```python
from build123d import *

# Parameters (mm, degrees)
SKETCH_1_W          = 6.2
SKETCH_1_H          = 6.2
SKETCH_1_R          = 1.2
EXTRUDE_1_DEPTH     = 2
CUT_EXTRUDE_1_DEPTH = 1
SKETCH_3_W          = 10
SKETCH_3_H          = 12.5
CUT_EXTRUDE_2_DEPTH = 1
CHAMFER_1_SIZE      = 1
SKETCH_4_W          = 44.4
SKETCH_4_H          = 18.5
SKETCH_4_W_2        = 38.4
SKETCH_4_H_2        = 12.5
EXTRUDE_2_DEPTH     = 3
CHAMFER_2_SIZE      = 2


with BuildPart() as part:
    # 草图1 → 凸台-拉伸1 (new body)
    with BuildSketch(Plane.XY):
        Polygon((-68.63, 16.2), (-64.63, 12.2), (-64.63, -37.62), (-68.63, -41.62), (-68.63, -49.62), (11.17, -49.62), (11.17, -41.62), (7.17, -37.62), (7.17, 12.2), (11.17, 16.2), (11.17, 38.1), (-68.63, 38.1), align=None)
        with Locations((-37.93, 28.38)):
            Rectangle(SKETCH_1_W, SKETCH_1_H, mode=Mode.SUBTRACT)
        with Locations((-27.73, 28.38)):
            Rectangle(SKETCH_1_W, SKETCH_1_H, mode=Mode.SUBTRACT)
        with Locations((-66.63, -45.62)):
            Circle(SKETCH_1_R, mode=Mode.SUBTRACT)
        with Locations((9.17, -45.62)):
            Circle(SKETCH_1_R, mode=Mode.SUBTRACT)
        with Locations((-66.63, 20.2)):
            Circle(SKETCH_1_R, mode=Mode.SUBTRACT)
        with Locations((9.17, 20.2)):
            Circle(SKETCH_1_R, mode=Mode.SUBTRACT)
    extrude(amount=EXTRUDE_1_DEPTH)

    # 草图2 → 切除-拉伸1 (cut)
    with BuildSketch(Plane.XY.offset(2)):
        Polygon((-12.23, -27.12), (-39.83, -27.12), (-39.83, -35.02), (-39.83, -39.62), (-12.23, -39.62), align=None)
        Polygon((-39.83, -27.12), (-50.63, -27.12), (-50.63, -39.62), (-39.83, -39.62), (-39.83, -35.02), align=None)
    extrude(amount=-CUT_EXTRUDE_1_DEPTH, mode=Mode.SUBTRACT)

    # 草图3 → 切除-拉伸2 (cut)
    with BuildSketch(Plane.XY.offset(1)):
        with Locations((-45.63, -33.37)):
            Rectangle(SKETCH_3_W, SKETCH_3_H)
    extrude(amount=-CUT_EXTRUDE_2_DEPTH, mode=Mode.SUBTRACT)

    # 倒角1
    chamfer_1_edges = [part.edges().sort_by_distance(p)[0] for p in [
        (-37.93, 25.28, 2),
        (-41.03, 28.38, 2),
        (-37.93, 31.48, 2),
        (-27.73, 31.48, 2),
        (-24.63, 28.38, 2),
        (-27.73, 25.28, 2),
        (-30.83, 28.38, 2),
        (-34.83, 28.38, 2),
    ]]
    chamfer(chamfer_1_edges, length=CHAMFER_1_SIZE)

    # 草图4 → 凸台-拉伸2 (add)
    with BuildSketch(Plane.XY.offset(2)):
        with Locations((-31.43, -33.37)):
            Rectangle(SKETCH_4_W, SKETCH_4_H)
        with Locations((-31.43, -33.37)):
            Rectangle(SKETCH_4_W_2, SKETCH_4_H_2, mode=Mode.SUBTRACT)
    extrude(amount=EXTRUDE_2_DEPTH)

    # 倒角2
    chamfer_2_edges = [part.edges().sort_by_distance(p)[0] for p in [
        (-31.43, -24.12, 5),
        (-9.23, -33.37, 5),
        (-53.63, -33.37, 5),
        (-31.43, -42.62, 5),
    ]]
    chamfer(chamfer_2_edges, length=CHAMFER_2_SIZE)


solid = part.part
```
Check sheet for the modelled part. Datum: model origin and axes. Units: mm. A direction names the side the tool comes from. Round coordinates to 2 decimals unless told otherwise and drop trailing zeros. Order: outer loops, then holes, each group sorted by start corner. A loop starts at its lowest first (then second) coordinate and runs counter-clockwise, first axis right, second up.
1) Go/stop test with flat-tipped pins: pin 1 Ø1 at (y, z) = (1, 4) entering from -X; pin 2 Ø1.6 at (y, z) = (-4.5, 1.5) entering from +X; pin 3 Ø0.5 at (x, z) = (-41, 2.5) entering from -Y; pin 4 Ø3 at (x, y) = (-66.63, 20.2) entering from +Z. Record where each tip stops, or that it passes through.
2) Section check A-A (y = -45.62). Record the boundary of the cut face in (x, z), and give its area (3 significant figures).
3) Scan lines: line 1 (Y direction, x = -21.5, z = 1.25); line 2 (Y direction, x = -66.63, z = 1.2); line 3 (X direction, y = -36.5, z = 0.35). Record each from-to range of solid material in increasing order.
4) Section check D-D (y = 26.5). Record the boundary of the cut face in (x, z).
5) Mould release check, pull along X, two halves, no side actions. Record for faces 1 (the cylindrical face through (9.724, -46.685, 0.986)), 2 (the flat face through (11.17, -46, 1)), 3 (the flat face through (-68.63, -46, 1)), 4 (the flat face through (-31.74, -25.11, 3.99)): +X half, -X half, draft (parallel to the pull), parting line (faces both ways), or undercut.
6) Section check B-B (x = -48). Record the boundary of the cut face in (y, z), and give its area (3 significant figures).
7) Section check C-C (x = -66.63). Record the boundary of the cut face in (y, z).
8) Tool access check on faces 5 (the flat face through (-64.63, -12, 1)), 6 (the flat face through (-27, -33, 1)), 7 (the flat face through (7.17, -13, 1)), 8 (the flat face through (-50.63, -33, 2)). Record the directions out of +Z, -Z, +X, -X, +Y, -Y that give a thin tool (end or side, any length) a straight path to the whole face; none if there is none.
Result:
1. pin 1: passes through
1. pin 2: stops at x = 7.17
1. pin 3: stops at y = -42.62
1. pin 4: stops at z = 2
2. outline: (-68.63, 0) - (-67.83, 0) - (-67.83, 2) - (-68.63, 2) - close; (-65.43, 0) - (7.97, 0) - (7.97, 2) - (-65.43, 2) - close; (10.37, 0) - (11.17, 0) - (11.17, 2) - (10.37, 2) - close
2. area: 150 mm2
3. line 1: y = -49.62 to -39.62, -27.12 to 38.1
3. line 2: y = -49.62 to -46.82, -44.42 to -39.62, 14.2 to 19, 21.4 to 38.1
3. line 3: x = -64.63 to -50.63, -40.63 to 7.17
4. outline: (-68.63, 0) - (-41.03, 0) - (-41.03, 1) - (-42.03, 2) - (-68.63, 2) - close; (-34.83, 0) - (-30.83, 0) - (-30.83, 1) - (-31.83, 2) - (-33.83, 2) - (-34.83, 1) - close; (-24.63, 0) - (11.17, 0) - (11.17, 2) - (-23.63, 2) - (-24.63, 1) - close
5. face 1: undercut
5. face 2: +X half
5. face 3: -X half
5. face 4: draft
6. outline: (-49.62, 0) - (-39.62, 0) - (-39.62, 5) - (-40.62, 5) - (-42.62, 3) - (-42.62, 2) - (-49.62, 2) - close; (-27.12, 0) - (38.1, 0) - (38.1, 2) - (-24.12, 2) - (-24.12, 3) - (-26.12, 5) - (-27.12, 5) - close
6. area: 164 mm2
7. outline: (-49.62, 0) - (-46.82, 0) - (-46.82, 2) - (-49.62, 2) - close; (-44.42, 0) - (-39.62, 0) - (-39.62, 2) - (-44.42, 2) - close; (14.2, 0) - (19, 0) - (19, 2) - (14.2, 2) - close; (21.4, 0) - (38.1, 0) - (38.1, 2) - (21.4, 2) - close
8. face 5: +Z, -Z, -X
8. face 6: +Z
8. face 7: +Z, -Z, +X
8. face 8: +Z, -Z
